Geometry: final body of the model. Coordinates: model frame, mm. A direction names the side the tool comes from. Give positions to 0.01 mm unless a question says otherwise; leave off trailing zeros. Loops run counter-clockwise (first coordinate to the right, second up) from the corner with the lowest first, then second, coordinate; pieces in that order, holes last. Notation, with made-up numbers: (72, 47) - (126, 47) arc R21 cw to (126, 73) - close; hole circle Ø5 at (-35.75, 3.5). An arc over 180 degrees is marked (long way). Use CSV: the item, a comma, the result in double quotes. Start each with the question number.
```python
from build123d import *

# Parameters (mm, degrees)
F0_W          = 8
F0_H          = 10
F1_DEPTH      = 8
F2_SIZE       = 4
F4_DEPTH      = 4
F5_DEPTH      = 3
F6_R          = 3.3
F7_DEPTH      = 3
F9_DEPTH      = 1.1
F11_R         = 1.9
F12_DEPTH     = 4
F13_R         = 2
F14_DEPTH     = 12.5
F15_T1_DEPTH  = 13.1433659759
F15_T6_DEPTH  = 13.1433659759
F15_S7_R      = 3
F15_T8_DEPTH  = 8
F16_W         = 1.5
F16_H         = 1.0667801354
F16_H_2       = 8
F16_H_3       = 0.8089432385
F17_DEPTH     = 1
F18_T4_DEPTH  = 11.5268513298
F18_S7_R      = 3.3
F18_T8_DEPTH  = 7
F18_T12_DEPTH = 11.5268513298
F18_S14_R     = 3.3
F18_T15_DEPTH = 7
F19_R         = 0.75
F20_DEPTH     = 25


# Not quite as in the source:
# - a fillet or chamfer that OpenCascade refuses, or shapes differently, is made with other operations: its cross-section is extruded or revolved along the edge and cut away or added


with BuildPart() as f1:
    # F0 (on Top) → F1 (new body)
    with BuildSketch(Plane.XY):
        with Locations((0, 5)):
            Rectangle(F0_W, F0_H)
    extrude(amount=F1_DEPTH)

    # F2
    f2_edges = [f1.edges().sort_by_distance(p)[0] for p in [
        (0, 0, 8),
        (0, 10, 8),
    ]]
    chamfer(f2_edges, length=F2_SIZE)

    # F3 (on Right) → F4 (join, symmetric)
    with BuildSketch(Plane.YZ):
        with BuildLine():
            ThreePointArc((2.1213203436, 6.1213203436), (-2.7716385975, 5.1480502971), (0, 1))
            Line((0, 1), (0, 4))
            Line((0, 4), (2.1213203436, 6.1213203436))
        make_face()
    extrude(amount=F4_DEPTH, both=True)

    # F3 (on Right) → F5 (join, symmetric)
    with BuildSketch(Plane.YZ):
        with BuildLine():
            Line((10, 4), (10, 1))
            ThreePointArc((10, 1), (12.1213203436, 1.8786796564), (13, 4))
            ThreePointArc((13, 4), (11.1480502971, 6.7716385975), (7.8786796564, 6.1213203436))
            Line((7.8786796564, 6.1213203436), (10, 4))
        make_face()
    extrude(amount=F5_DEPTH, both=True)

    # F6 (on Right) → F7 (cut, symmetric)
    with BuildSketch(Plane.YZ):
        with Locations((0, 4.1532493821)):
            Circle(F6_R)
    extrude(amount=F7_DEPTH, both=True, mode=Mode.SUBTRACT)

    # F8 (on face) → F9 (cut)
    with BuildSketch(Plane(origin=(-4, 0, 0), x_dir=(0, -1, 0), z_dir=(-1, 0, 0))):
        with BuildLine():
            Line((-10, 4), (-7.7019029611, 6.2980970389))
            ThreePointArc((-7.7019029611, 6.2980970389), (-13.0026084807, 5.2437211552), (-10, 0.75))
            Line((-10, 0.75), (-10, 4))
        make_face()
        with BuildLine():
            ThreePointArc((-10, 0.75), (-7.7019029611, 1.7019029611), (-6.75, 4))
            ThreePointArc((-6.75, 4), (-6.9973915193, 5.2437211552), (-7.7019029611, 6.2980970389))
            Line((-7.7019029611, 6.2980970389), (-10, 4))
            Line((-10, 4), (-10, 0.75))
        make_face()
    extrude(amount=-F9_DEPTH, mode=Mode.SUBTRACT)

    # F10: F1 across plane


with BuildPart() as f1_1:
    add(f1.part)
    add(f1.part.mirror(Plane.YZ), mode=Mode.INTERSECT)

    # F11 (on Right) → F12 (join, symmetric)
    with BuildSketch(Plane.YZ):
        with Locations((10, 4)):
            Circle(F11_R)
    extrude(amount=F12_DEPTH, both=True)

    # F13 (on Right) → F14 (cut, symmetric)
    with BuildSketch(Plane.YZ):
        with Locations((0, 4)):
            Circle(F13_R)
    extrude(amount=F14_DEPTH, both=True, mode=Mode.SUBTRACT)

    # F15: chamfer of 1 on 2 edges, made by hand

    # F15_s2 → F15_t1 (cut)
    with BuildSketch(Plane.YZ.offset(-6.571682988)):
        Polygon((1, 0), (0, 1), (0, 0), align=None)
    extrude(amount=F15_T1_DEPTH, mode=Mode.SUBTRACT)


with BuildPart() as f15_tool4:
    # F15_s5 → F15_t6 (new body)
    with BuildSketch(Plane.YZ.offset(6.571682988)):
        Polygon((9, 0), (10, 1), (10, 0), align=None)
    extrude(amount=-F15_T6_DEPTH)

    # F15_s7 → F15_t8 (cut, symmetric)
    with BuildSketch(Plane.YZ):
        with Locations((10, 4)):
            Circle(F15_S7_R)
    extrude(amount=F15_T8_DEPTH, both=True, mode=Mode.SUBTRACT)


with BuildPart() as f1_2:
    add(f1_1.part)

    # F15_t3: cut F15_tool4
    add(f15_tool4.part, mode=Mode.SUBTRACT)

    # F16 (on face) → F17 (cut)
    with BuildSketch(Plane(origin=(0, 0, 0), x_dir=(1, 0, 0), z_dir=(0, 0, -1))):
        with Locations((0, -9.5333900677)):
            Rectangle(F16_W, F16_H)
        with Locations((0, -5)):
            Rectangle(F16_W, F16_H_2)
        with Locations((0, -0.5955283808)):
            Rectangle(F16_W, F16_H_3)
    extrude(amount=-F17_DEPTH, mode=Mode.SUBTRACT)

    # F18: fillet of radius 0.5 on 2 edges, made by hand


with BuildPart() as f18_tool2:
    # F18_s3 → F18_t4 (new body)
    with BuildSketch(Plane.XZ.offset(0.2768513298)):
        with BuildLine():
            ThreePointArc((-0.75, 0.5), (-0.6035533906, 0.8535533906), (-0.25, 1))
            Line((-0.25, 1), (-0.75, 1))
            Line((-0.75, 1), (-0.75, 0.5))
        make_face()
    extrude(amount=-F18_T4_DEPTH)

    split(bisect_by=Plane(origin=(0, 0.5, 0.5), x_dir=(1, 0, 0), z_dir=(0, 0.7071067812, 0.7071067812)), keep=Keep.TOP)

    split(bisect_by=Plane(origin=(0, 4.5, -4.5), x_dir=(1, 0, 0), z_dir=(0, -0.7071067812, 0.7071067812)), keep=Keep.TOP)

    # F18_s7 → F18_t8 (cut, symmetric)
    with BuildSketch(Plane.YZ.offset(-0.5)):
        with Locations((0, 4.1532493821)):
            Circle(F18_S7_R)
    extrude(amount=F18_T8_DEPTH, both=True, mode=Mode.SUBTRACT)


with BuildPart() as f1_3:
    add(f1_2.part)

    # F18_t1: union F18_tool2
    add(f18_tool2.part)


with BuildPart() as f18_tool10:
    # F18_s11 → F18_t12 (new body)
    with BuildSketch(Plane.XZ.offset(-11.25)):
        with BuildLine():
            ThreePointArc((0.75, 0.5), (0.6035533906, 0.8535533906), (0.25, 1))
            Line((0.25, 1), (0.75, 1))
            Line((0.75, 1), (0.75, 0.5))
        make_face()
    extrude(amount=F18_T12_DEPTH)

    split(bisect_by=Plane(origin=(0, 0.5, 0.5), x_dir=(1, 0, 0), z_dir=(0, 0.7071067812, 0.7071067812)), keep=Keep.TOP)

    # F18_s14 → F18_t15 (cut, symmetric)
    with BuildSketch(Plane.YZ.offset(0.5)):
        with Locations((0, 4.1532493821)):
            Circle(F18_S14_R)
    extrude(amount=F18_T15_DEPTH, both=True, mode=Mode.SUBTRACT)

    split(bisect_by=Plane(origin=(0, 4.5, -4.5), x_dir=(1, 0, 0), z_dir=(0, -0.7071067812, 0.7071067812)), keep=Keep.TOP)


with BuildPart() as f1_4:
    add(f1_3.part)

    # F18_t9: union F18_tool10
    add(f18_tool10.part)

    # F19 (on Front) → F20 (cut)
    with BuildSketch(Plane.XZ):
        with Locations((0, 6.8)):
            Circle(F19_R)
    extrude(amount=-F20_DEPTH, mode=Mode.SUBTRACT)


solid = f1_4.part
```
Item 1: Section C-C (z = 4.25). Output: boundary loops of the cut face in (x, y).
Item 2: Section B-B (y = -1.5). Output: boundary loops of the cut face in (x, z).
Item 3: Reachability of faces 1 (the flat face through (3, 2, 3)), 2 (the flat face through (-2.9, 8.5, 2.5)), 3 (the flat face through (0, 5, 8)) from +Z, -Z, +X, -X, +Y, -Y: full face, straight path, thin tool, end or side. Return the list, or none.
Item 4: Mould query, pull axis Z, two halves, no side actions, for faces 4 (the flat face through (-0.1, 6.3, 7.7)), 5 (the flat face through (-4, 10, 4)), 6 (the cylindrical face through (-3.442, 11.021, 5.602)). Classes: pulls with the +Z half, pulls with the -Z half, needs draft (parallel to the pull), parting line crosses it, or undercut.
Item 5: Pin query (flat end, axial travel): pin 1 Ø3 at (y, z) = (0, 4) entering from +X. Return the tip coordinate at first contact, or that it passes through.
Item 6: Section D-D (z = 7.25). Output: boundary loops of the cut face in (x, y), plus the area to 3 significant figures.
Item 7: Ray query, probe 1 along X at (y, z) = (2, 3.25); probe 2 along Z at (x, y) = (0, 5); probe 3 along X at (y, z) = (4, 6.75). Return the intervals inside material, ascending.
Item 8: Section A-A (x = -3.25). Output: boundary loops of the cut face in (y, z), plus the area to 3 significant figures.
Outcome:
1,outline,"(-4, -2.99) - (-3, -2.99) - (-3, -1.98) - (-4, -1.98) - close; (-4, 1.98) - (-3, 1.98) - (-3, 3.3) - (3, 3.3) - (3, 1.98) - (4, 1.98) - (4, 6.76) - (2.9, 6.76) - (2.9, 8.12) - (4, 8.12) - (4, 11.88) - (2.9, 11.88) - (2.9, 12.99) - (-2.9, 12.99) - (-2.9, 11.88) - (-4, 11.88) - (-4, 8.12) - (-2.9, 8.12) - (-2.9, 6.76) - (-4, 6.76) - close; (3, -2.99) - (4, -2.99) - (4, -1.98) - (3, -1.98) - close"
2,outline,"(-4, 1.4) - (-3, 1.4) - (-3, 2.68) - (-4, 2.68) - close; (-4, 5.32) - (-3, 5.32) - (-3, 6.6) - (-4, 6.6) - close; (3, 1.4) - (4, 1.4) - (4, 2.68) - (3, 2.68) - close; (3, 5.32) - (4, 5.32) - (4, 6.6) - (3, 6.6) - close"
3,face 1,"-Y"
3,face 2,"-X"
3,face 3,"+Z, +X, -X, +Y, -Y"
4,face 4,"pulls with the +Z half"
4,face 5,"needs draft"
4,face 6,"undercut"
5,pin 1,"passes through"
6,outline,"(-4, 3.25) - (-0.6, 3.25) - (-0.6, 6.75) - (-4, 6.75) - close; (0.6, 3.25) - (4, 3.25) - (4, 6.75) - (0.6, 6.75) - close"
6,area,"23.8 mm2"
7,probe 1,"x = -4 to -3, 3 to 4"
7,probe 2,"z = 1 to 6.05, 7.55 to 8"
7,probe 3,"x = -4 to -0.75, 0.75 to 4"
8,outline,"(0, 1) - (1, 0) - (9, 0) - (9.76, 0.76) arc R3.25 cw to (7.7, 6.3) - (6, 8) - (4, 8) - (2.12, 6.12) arc R3 ccw (long way) to start; circle Ø3.8 at (10, 4); hole circle Ø4 at (0, 4)"
8,area,"67.0 mm2"
